Autodesk Inventor part; units mm, degrees
ref_plane "YZ Plane" through (0, 0, 0) normal (1, 0, 0) x (0, 1, 0)
ref_plane "XZ Plane" through (0, 0, 0) normal (0, 1, 0) x (-1, 0, 0)
ref_plane "XY Plane" through (0, 0, 0) normal (0, 0, 1) x (1, 0, 0)
sketch "Sketch2" plane through (0, 0, 0) normal (1, 0, 0) x (0, 1, 0)
  line L0 (0, 0) -> (20, 0)
  line L1 (30, 10) -> (-10, 10)
  line L2 (-10, 20) -> (-10, 10)
  line L3 (30, 20) -> (30, 10)
  line L4 (20, 0) -> (30, 10)
  line L5 (0, 0) -> (-10, 10)
  line L6 (10, 0) -> (10, 7) construction
  circle A0 centre (10, 7) radius 2.5
  circle A1 centre (10, 7) radius 8 construction
  line L7 (-10, 20) -> (30, 20)
  arc A2 (18.4853, 10) -> (1.5147, 10) centre (10, 7) ccw
  point P0 (10, 10)
  point P1 (1.9377, 11)
  dimension "d12" = 10
  dimension "d15" = 45
  dimension "d16" = 20
  dimension "d17" = 7
  dimension "d18" = 5
  dimension "d19" = 16
  dimension "square_thickness" = 10
  dimension "d22" = 9
  dimension "d55" = 11
extrude "Extrusion1" add sketch "Sketch2" along normal blind 5 contours L5 L1 L4 L0
extrude "Extrusion2" add sketch "Sketch2" against normal blind 6 contours L2 L7 L3 L1 A2
extrude "Extrusion3" add sketch "Sketch2" against normal blind 5 from surface at -6 contours L5 L1 L4 L0
extrude "Extrusion4" add sketch "Sketch2" along normal blind 23 contours L2 L7 L3 L1 A2 | A2 L1
extrude "Extrusion5" add sketch "Sketch2" against normal blind 23 from surface at -6 contours L2 L7 L3 L1 A2 | A2 L1
sketch "Sketch4" plane through (23, 30, 10) normal (0, 0, -1) x (-1, 0, 0)
  line L0 (52, -40) -> (52, 0) construction
  line L1 (52, -20) -> (0, -20) construction
  line L2 (0, 0) -> (0, -40) construction
  circle A0 centre (4, -20) radius 2
  line L3 (0, -40) -> (0, 0) construction
  circle A1 centre (48, -20) radius 2
  line L4 (52, 0) -> (52, -40) construction
  point P0 (23, -30)
  dimension "d39" = 4
  dimension "d40" = 4
  dimension "d41" = 4
  dimension "d42" = 4
hole "Hole1" at (19, 10, 10) at (-25, 10, 10) direction (0, 0, 1) diameter 4 end through all counterbore diameter 6 counterbore depth 2
sketch "Sketch5" plane through (-6, 30, 10) normal (0, 1, 0) x (1, 0, 0)
  line L0 (-23, -10) -> (-23, 0)
  line L1 (-23, 0) -> (-33, -10)
  line L2 (-33, -10) -> (-23, -10)
  line L3 (-23, -10) -> (29, -10)
  line L4 (29, -10) -> (39, -10)
  line L5 (29, 0) -> (29, -10)
  line L6 (39, -10) -> (29, 0)
  point P0 (6, 10)
  dimension "d51" = 45
  dimension "d52" = 45
extrude "Extrusion6" add sketch "Sketch5" against normal up to surface (40 mm away)
equation "\"d18\" = ball_bearing_ID"
equation "\"d19\" = ball_bearing_OD"
equation "\"d33\" = d29"
equation "\"d40\" = screw_size"
equation "\"d41\" = screw_size"
equation "\"d43\" = screw_size"
equation "\"ball_bearing_ID\" = 5"
equation "\"ball_bearing_OD\" = 16"
equation "\"ball_bearing_width\" = 5"
equation "\"screw_size\" = 4"
properties part number "3_inner_glider_carriage"
The model under review builds one solid part; all positions refer to its coordinate system, in mm. A direction names the side the tool comes from. Give positions to 0.01 mm unless a question says otherwise; leave off trailing zeros. Order: outer loops, then holes, each group sorted by start corner. A loop starts at its lowest first (then second) coordinate and runs counter-clockwise, first axis right, second up. Notation, with made-up numbers: M 29,56.25 L 36,56.25 A18 cw 36,77.25 Z; hole C 19.5,-10 d6. An arc over 180 degrees is marked long. One line per question, with ' | ' between items. Start each with the question number.
1) Mouldability with a two-part tool opening along X and no side actions: class faces 1 (the face through (-3, 24, 10)), 2 (the face through (-34, 10, 15)), 3 (the face through (28, 10, 15)), 4 (the face through (-20, 10, 10)) as pulls with the +X half, pulls with the -X half, needs draft (parallel to the pull), parting line crosses it, or undercut.
2) Consider section C-C, the plane y = -6. Give the boundary of the cut face in (x, z), then the cut area to 3 significant figures.
3) Consider section D-D, the plane z = 12.75. Give the boundary of the cut face in (x, y), then the cut area to 3 significant figures.
4) Consider section B-B, the plane x = -25. Give the boundary of the cut face in (y, z), then the cut area to 3 significant figures.
5) For faces 5 (the face through (14, 10, 10)), 6 (the face through (-23.85, 12.77, 11.01)), 7 (the face through (-2, -10, 15)), list the 3-axis set-ups (+Z, -Z, +X, -X, +Y, -Y) from which the entire face can be reached by the end or side of a thin tool; tool diameter is ignored.
6) Clearance check with flat-ended pins moving along their axes: P1, Ø2, axis at x = -25, y = 21, coming from the -Z side; P2, Ø11, axis at y = 18.5, z = 6.5, coming from the +X side; P3, Ø1, axis at y = 6, z = 5.5, coming from the +X side. State where each tip first meets the part, or that it passes through.
7) Wall thickness on L1, parallel to Z at x = 2.55, y = 10; L2, parallel to X at y = 10, z = 10.5; L3, parallel to X at y = 1, z = 7.25: over which ranges is each line inside the solid? List them lowest first. Write a range as from..to.
8) Consider section A-A, the plane z = 7. Give the boundary of the cut face in (x, y), then the cut area to 3 significant figures.
Found:
1) face 1: undercut | face 2: pulls with the -X half | face 3: pulls with the +X half | face 4: needs draft
2) outline: M -39,20 L -29,10 L -11,10 L -11,6 L -6,6 L -6,10 L 0,10 L 0,6 L 5,6 L 5,10 L 23,10 L 33,20 Z | area: 660 mm²
3) outline: M -31.75,-10 L 25.75,-10 L 25.75,30 L -31.75,30 Z; hole C -25,10 d4; hole M -6,3.08 L 0,3.08 L 0,16.92 L -6,16.92 Z; hole C 19,10 d4 | area: 2,190 mm²
4) outline: M -10,10 L 7,10 L 7,12 L 8,12 L 8,20 L -10,20 Z; M 12,12 L 13,12 L 13,10 L 30,10 L 30,20 L 12,20 Z | area: 356 mm²
5) face 5: -Z, +X, +Y, -Y | face 6: -Z | face 7: +Z, -Z, +X, -X, -Y
6) P1: stops at z = 10 | P2: stops at x = 25 | P3: stops at x = 5
7) L1: z = 0..4.5, 9.5..20 | L2: x = -29.5..-28, -22..-6, 0..16, 22..23.5 | L3: x = -11..-6, 0..5
8) outline: M -11,-7 L -6,-7 L -6,7.5 L -11,7.5 Z; M -11,12.5 L -6,12.5 L -6,27 L -11,27 Z; M 0,-7 L 5,-7 L 5,7.5 L 0,7.5 Z; M 0,12.5 L 5,12.5 L 5,27 L 0,27 Z | area: 290 mm²
